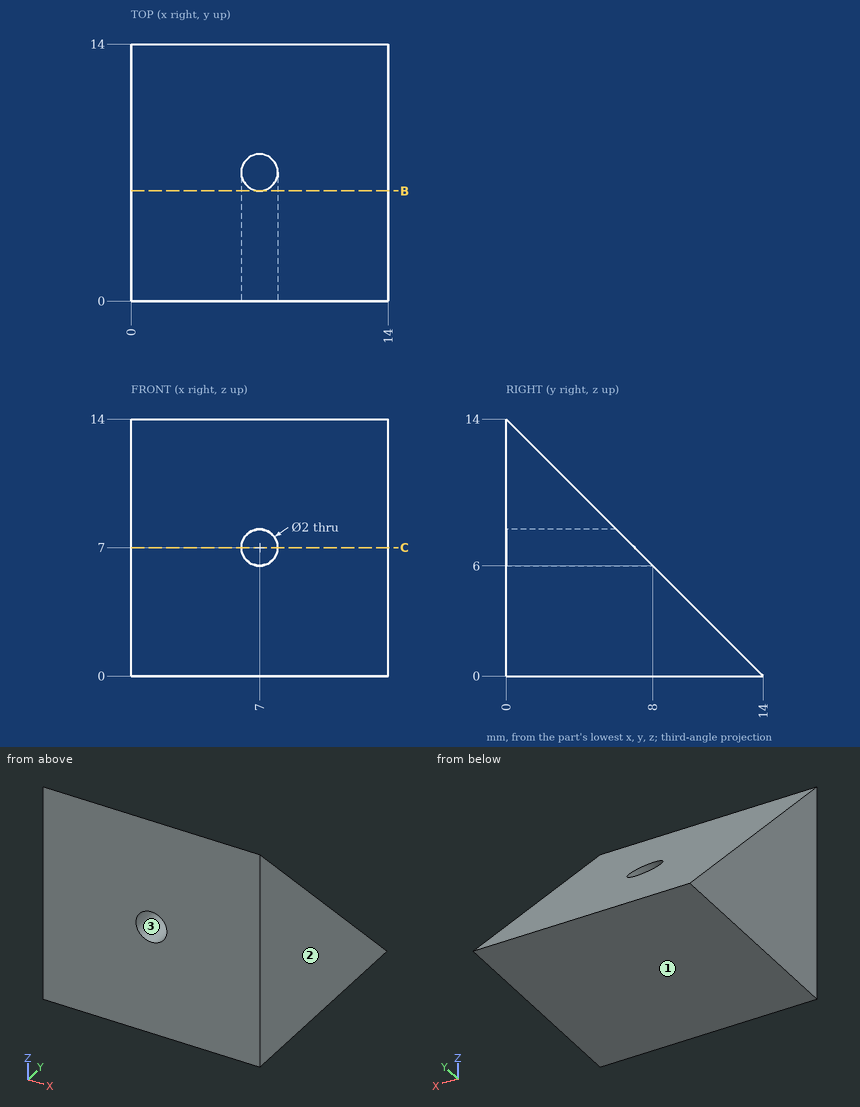
The figure shows three views and two pictorial views of one solid part (mm, origin at its lowest corner). Answer the questions. Coordinates: 2 decimals unless noted, no trailing zeros. Write each loop counter-clockwise with the first axis right and the second up, starting at its lowest first coordinate (ties: lowest second). Pieces come first, ordered by that corner, then holes. Notation, with made-up numbers: (20.5, -7) -> (77.5, -7) arc R28 cw to (77.5, 20) -> close; hole circle Ø1 at (33, -12). An arc over 180 degrees is marked (long way). Answer as a JSON object with one key per item and string values.
Q1. Flat-ended cylindrical pins translate along their axes: pin 1 Ø1 at (x, z) = (10.5, 11.5) entering from +Y; pin 2 Ø8 at (x, z) = (2, 10) entering from +Y; pin 3 Ø5 at (x, y) = (6, 9.5) entering from +Z. Find the tip coordinate at first contact, or state that the pin passes through.
The answers:
{"pin 1": "stops at y = 3", "pin 2": "stops at y = 8", "pin 3": "stops at z = 7"}
Q2. The part is cut by section B-B on y = 6. Give the vertices of the cut face in (x, z).
The answers:
{"outline": "(0, 0) -> (14, 0) -> (14, 8) -> (0, 8) -> close; hole circle Ø2 at (7, 7)"}
Q3. Determine the mould class of the marked faces 1, 2 and 3 for opening direction X: pulls with the +X half, pulls with the -X half, needs draft (parallel to the pull), parting line crosses it, or undercut.
The answers:
{"face 1": "needs draft", "face 2": "pulls with the +X half", "face 3": "undercut"}
Q4. The part is cut by section C-C on z = 7. Give the vertices of the cut face in (x, y), then the cut area to 3 significant figures.
The answers:
{"outline": "(0, 0) -> (6, 0) -> (6, 7) -> (0, 7) -> close; (8, 0) -> (14, 0) -> (14, 7) -> (8, 7) -> close", "area": "84.0 mm2"}
Q5. Consider line 1 (X direction, y = 4.25, z = 7); line 2 (Z direction, x = 7, y = 2); line 3 (Z direction, x = 7, y = 3.25). Determine where each line is inside the solid, lowest interval first. Write a range as [from, to].
The answers:
{"line 1": "x = [0, 6], [8, 14]", "line 2": "z = [0, 6], [8, 12]", "line 3": "z = [0, 6], [8, 10.75]"}
